Source: CAD feature listing. Evaluate the final solid. Frame: model axes, mm. A direction names the side the tool comes from. Round coordinates to 2 decimals unless told otherwise and drop trailing zeros. Write each loop counter-clockwise with the first axis right and the second up, starting at its lowest first coordinate (ties: lowest second). Pieces come first, ordered by that corner, then holes.
from build123d import *

# Parameters (mm, degrees)
F2_W     = 5.9578604996
F2_H     = 4.390229471
F3_DEPTH = 19.05


# Not quite as in the source:
# - the program builds the solid bodies; features that only make, move or delete a surface that nothing else refers to are left out


with BuildPart() as f3:
    # F2 (on Top) → F3 (new body)
    with BuildSketch(Plane.XY):
        Polygon((48.7568192184, 33.4314107895), (38.8487800956, 33.4314107895), (38.8487800956, 29.4627081603), (38.8487800956, 12.5663736835), (38.8487800956, 8.1761442125), (48.7568192184, 8.1761442125), align=None)
        Polygon((38.8487800956, 29.4627081603), (38.8487800956, 33.4314107895), (38.8487800956, 33.7930396199), (32.8023135662, 33.7930396199), (32.8023135662, 29.4627081603), align=None)
        with Locations((35.8698498458, 10.371258948)):
            Rectangle(F2_W, F2_H)
    extrude(amount=F3_DEPTH)


solid = f3.part
1) Section query A-A on x = 35.5. Return the cut outline in (y, z), then the cut area to 3 significant figures.
Taken from the geometry:
outline: (8.18, 0) - (12.57, 0) - (12.57, 19.05) - (8.18, 19.05) - close; (29.46, 0) - (33.79, 0) - (33.79, 19.05) - (29.46, 19.05) - close
area: 166 mm2
2) Section query B-B on z = 13.75. Return the cut outline in (x, y).
Taken from the geometry:
outline: (32.8, 29.46) - (38.85, 29.46) - (38.85, 12.57) - (32.89, 12.57) - (32.89, 8.18) - (48.76, 8.18) - (48.76, 33.43) - (38.85, 33.43) - (38.85, 33.79) - (32.8, 33.79) - close
3) Pull-direction query (Y, two-part tool) for faces 4 (the face through (36, 12.566, 9)), 5 (the face through (36, 29.463, 9)), 6 (the face through (44, 33.431, 9)), 7 (the face through (48.757, 21, 9)); classes: released by +Y, released by -Y, zero draft, split by the parting line, or undercut.
Taken from the geometry:
face 4: undercut
face 5: undercut
face 6: released by +Y
face 7: zero draft
4) Contact query for flat-ended pins moving along their axis: P1, Ø8.5, axis at y = 21.5, z = 8, coming from the -X side; P2, Ø8, axis at x = 46, z = 6, coming from the +Y side; P3, Ø1, axis at y = 10.5, z = 8.5, coming from the -X side; P4, Ø5, axis at y = 28, z = 13.5, coming from the -X side. Output: stop coordinate, or through.
Taken from the geometry:
P1: stops at x = 38.85
P2: stops at y = 33.43
P3: stops at x = 32.89
P4: stops at x = 32.8
5) Section query C-C on y = 25.75. Return the cut outline in (x, z).
Taken from the geometry:
outline: (38.85, 0) - (48.76, 0) - (48.76, 19.05) - (38.85, 19.05) - close
6) Material intervals for line 1 (Y direction, x = 34.25, z = 5); line 2 (Y direction, x = 45.25, z = 1.5); line 3 (X direction, y = 21, z = 5.25), sorted ascending.
Taken from the geometry:
line 1: y = 8.18 to 12.57, 29.46 to 33.79
line 2: y = 8.18 to 33.43
line 3: x = 38.85 to 48.76
7) Reachability of faces 1 (the face through (38.849, 21, 9)), 2 (the face through (42, 21, 0)), 3 (the face through (32.891, 10, 9)) from +Z, -Z, +X, -X, +Y, -Y: full face, straight path, thin tool, end or side. Return the list, or none.
Taken from the geometry:
face 1: +Z, -Z, -X
face 2: -Z, +X, -X, +Y, -Y
face 3: +Z, -Z, -X, -Y
